For this review, use the dimensioned drawing (mm, ordinates from the lowest corner) and the shaded views. A direction names the side the tool comes from. Coordinates: 2 decimals unless noted, no trailing zeros. Loops run counter-clockwise (first coordinate to the right, second up) from the corner with the lowest first, then second, coordinate; pieces in that order, holes last. Notation, with made-up numbers: (39.25, 85.25) - (72.25, 85.25) arc R10 cw to (72.25, 98.25) - close; hole circle Ø1 at (46, -37.5). An arc over 180 degrees is marked (long way). Use a Markdown table: item, result. Add a question column.
1) Add section C-C, the plane x = 38. Give the boundary of the cut face in (y, z), and give its area (3 significant figures).
2) Clearance check with flat-ended pins moving along their axes: pin 1 (12 mm diameter, centred on x = 60, y = 15.5, fed in from -Z); pin 2 (10 mm diameter, centred on x = 40, y = 8.5, fed in from +Z) (1 decimal); pin 3 (2 mm diameter, centred on y = 28, z = 70, fed in from -X); pin 4 (12 mm diameter, centred on y = 24.5, z = 71, fed in from +X) (1 decimal). State where each tip first meets the part, or that it passes through.
3) Add section D-D, the plane y = 55. Give the boundary of the cut face in (x, z) (1 decimal).
4) Add section B-B, the plane x = 78. Give the boundary of the cut face in (y, z) (1 decimal).
5) For the marked faces 1 and 2, list the 3-axis set-ups (+Z, -Z, +X, -X, +Y, -Y) from which the entire face can be reached by the end or side of a thin tool; tool diameter is ignored.
6) Add section A-A, the plane z = 57. Give the boundary of the cut face in (x, y) (1 decimal).
7) To check wall thickness, follow L1, parallel to Y at x = 19.5, z = 24.5; L2, parallel to Z at x = 80.5, y = 61 (1 decimal); L3, parallel to Z at x = 60, y = 26.5 (1 decimal). State the ranges of each line that lie inside material, in increasing order. Write a range as [from, to].
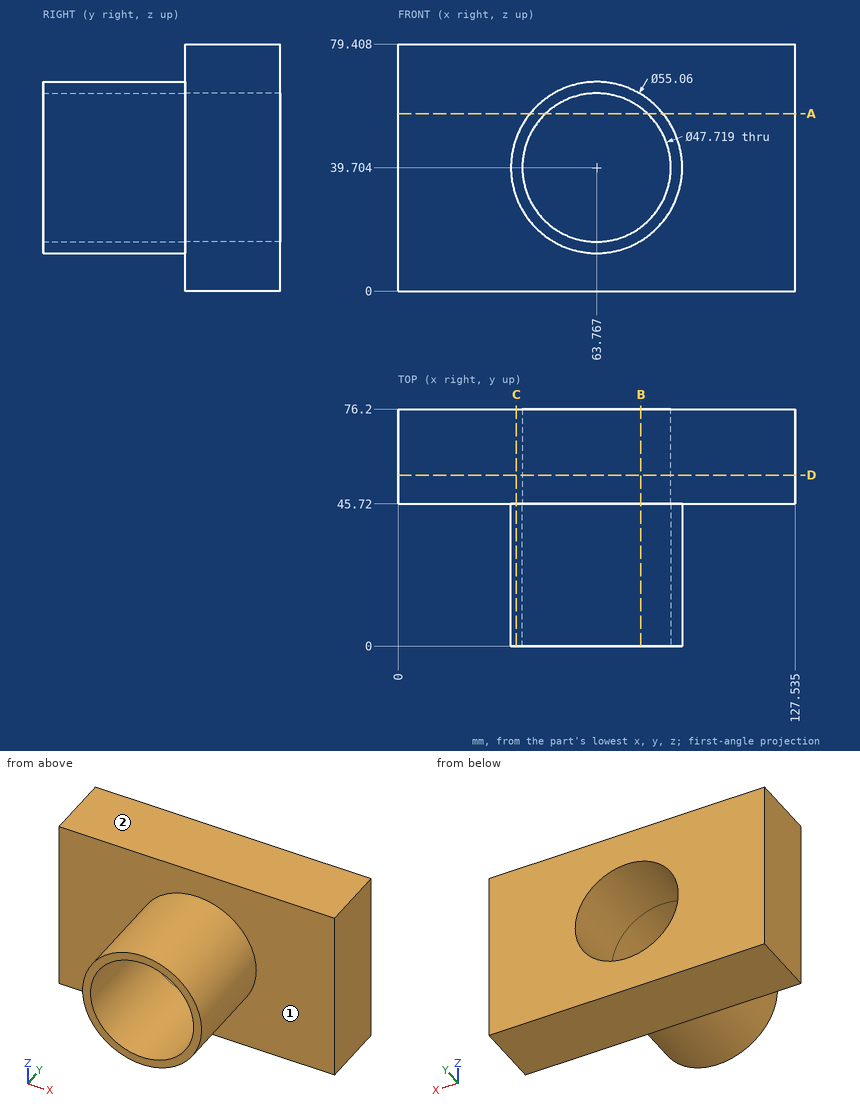
From the geometry:
| question | item | result |
|---|---|---|
| 1 | outline | (0, 30.01) - (45.72, 30.01) - (45.72, 0) - (76.2, 0) - (76.2, 79.41) - (45.72, 79.41) - (45.72, 49.4) - (0, 49.4) - close |
| 1 | area | 3,310 mm^2 |
| 2 | pin 1 | stops at z = 12.17 |
| 2 | pin 2 | stops at z = 59.8 |
| 2 | pin 3 | passes through |
| 2 | pin 4 | stops at x = 74.6 |
| 3 | outline | (0, 0) - (127.5, 0) - (127.5, 79.4) - (0, 79.4) - close; hole circle Ø47.7 at (63.8, 39.7) |
| 4 | outline | (0, 16.1) - (45.7, 16.1) - (45.7, 0) - (76.2, 0) - (76.2, 20.6) - (0, 20.6) - close; (0, 58.9) - (76.2, 58.9) - (76.2, 79.4) - (45.7, 79.4) - (45.7, 63.3) - (0, 63.3) - close |
| 5 | face 1 | -Y |
| 5 | face 2 | +Z, +X, -X, +Y, -Y |
| 6 | outline | (0, 45.7) - (42.3, 45.7) - (42.3, 0) - (47.3, 0) - (47.3, 76.2) - (0, 76.2) - close; (80.2, 0) - (85.2, 0) - (85.2, 45.7) - (127.5, 45.7) - (127.5, 76.2) - (80.2, 76.2) - close |
| 7 | L1 | y = [45.72, 76.2] |
| 7 | L2 | z = [0, 22.7], [56.7, 79.4] |
| 7 | L3 | z = [12.4, 16.1], [63.3, 67] |
